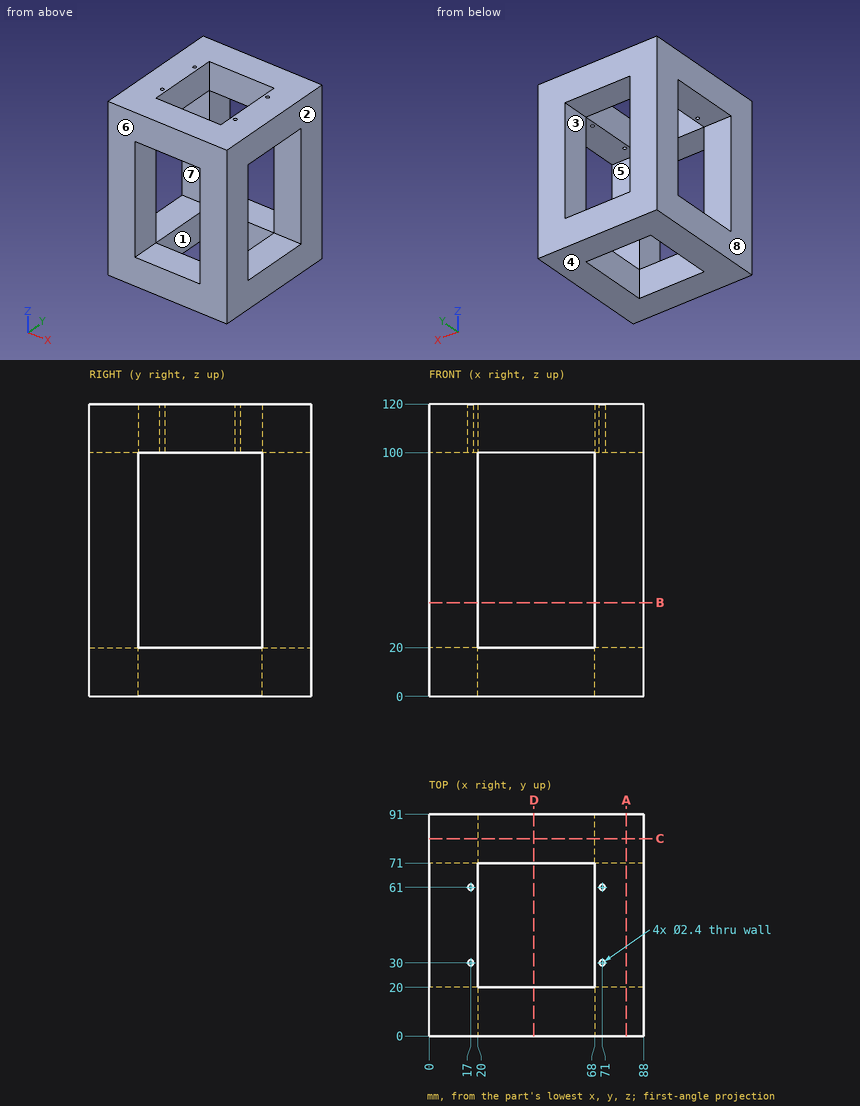
Answer from the drawing. Dimensions are ordinates in mm from the lowest x, y and z of the part. A direction names the side the tool comes from. Give positions to 0.01 mm unless a question says otherwise; leave off trailing zeros. Order: outer loops, then holes, each group sorted by start corner. A loop starts at its lowest first (then second) coordinate and runs counter-clockwise, first axis right, second up. Notation, with made-up numbers: (1, 55.5) - (20, 55.5) arc R23 ccw to (20, 68.5) - close; hole circle Ø1 at (84.25, 70). An arc over 180 degrees is marked (long way). One line per item, written item: value. Start each with the question number.
1. Section D-D, the plane x = 43 is taken. Write down the section's boundary in (y, z), then the cut area to 3 significant figures.
2. Consider line 1 (Y direction, x = 10, z = 82.5); line 2 (X direction, y = 70.5, z = 10.5); line 3 (Z direction, x = 58, y = 77.5). Determine where each line is inside the solid, lowest interval first.
3. Section A-A, the plane x = 81 is taken. Write down the section's boundary in (y, z), then the cut area to 3 significant figures.
4. For a pull along Y with two mould halves and no side action, classify the marked faces 6, 7 and 8 as released by +Y, released by -Y, zero draft, split by the parting line, or undercut.
5. Section C-C, the plane y = 81 is taken. Write down the section's boundary in (x, z).
6. Which of the six approach directions +Z, -Z, +X, -X, +Y, -Y give full straight-line access (tool end or side, diameter ignored) to the marked faces 1, 2, 3, 4 and 5?
7. Each of these flat-tipped pins is pushed along its axis until it touches: pin 1 Ø2 at (x, y) = (17, 61) entering from +Z; pin 2 Ø4 at (x, y) = (64.5, 47) entering from -Z. Where does it stop, or does it pass through?
8. Section B-B, the plane z = 38.5 is taken. Write down the section's boundary in (x, y).
Filled sheet:
1. outline: (0, 0) - (20, 0) - (20, 20) - (0, 20) - close; (0, 100) - (20, 100) - (20, 120) - (0, 120) - close; (71, 0) - (91, 0) - (91, 20) - (71, 20) - close; (71, 100) - (91, 100) - (91, 120) - (71, 120) - close
1. area: 1,600 mm²
2. line 1: 0 to 20, 71 to 91
2. line 2: 0 to 20, 68 to 88
2. line 3: 0 to 20, 100 to 120
3. outline: (0, 0) - (91, 0) - (91, 120) - (0, 120) - close; hole (20, 20) - (71, 20) - (71, 100) - (20, 100) - close
3. area: 6,840 mm²
4. face 6: released by -Y
4. face 7: undercut
4. face 8: zero draft
5. outline: (0, 0) - (88, 0) - (88, 120) - (0, 120) - close; hole (20, 20) - (68, 20) - (68, 100) - (20, 100) - close
6. face 1: +Z, -Z
6. face 2: +Z, -Z, +X, +Y, -Y
6. face 3: +Y, -Y
6. face 4: -Z, +X, -X, +Y, -Y
6. face 5: +X, -X
7. pin 1: z = 20
7. pin 2: through
8. outline: (0, 0) - (20, 0) - (20, 20) - (0, 20) - close; (0, 71) - (20, 71) - (20, 91) - (0, 91) - close; (68, 0) - (88, 0) - (88, 20) - (68, 20) - close; (68, 71) - (88, 71) - (88, 91) - (68, 91) - close
